```python
from build123d import *

# Parameters (mm, degrees)
ESBO_O1_W                = 120
ESBO_O1_H                = 204
RESSALTO_EXTRUS_O1_DEPTH = 60
ESBO_O2_W                = 114
ESBO_O2_H                = 198
CORTE_EXTRUS_O1_DEPTH    = 57
ESBO_O4_W                = 86
ESBO_O4_H                = 149
CORTE_EXTRUS_O2_DEPTH    = 45
ESBO_O7_W                = 3
ESBO_O7_H                = 204
RESSALTO_EXTRUS_O2_DEPTH = 15
ESBO_O12_W               = 3
ESBO_O12_H               = 204
RESSALTO_EXTRUS_O3_DEPTH = 15
ESBO_O13_W               = 150
ESBO_O13_H               = 3
RESSALTO_EXTRUS_O4_DEPTH = 10
ESBO_O14_W               = 150
ESBO_O14_H               = 3
RESSALTO_EXTRUS_O5_DEPTH = 10
FILETE1_R                = 10
ESBO_O15_W               = 3
ESBO_O15_H               = 5
ESBO_O15_W_2             = 5
ESBO_O15_H_2             = 3
CORTE_EXTRUS_O4_DEPTH    = 5
FILETE2_R                = 10
FILETE3_R                = 10
FILETE4_R                = 10
FILETE5_R                = 2
FILETE6_R                = 2
FILETE8_R                = 2


with BuildPart() as part:
    # Esboço1 → Ressalto-extrusão1 (new body)
    with BuildSketch(Plane.XY):
        with Locations((27.324641181, 48.820153307)):
            Rectangle(ESBO_O1_W, ESBO_O1_H)
    extrude(amount=RESSALTO_EXTRUS_O1_DEPTH)

    # Esboço2 → Corte-extrusão1 (cut)
    with BuildSketch(Plane(origin=(0, 0, 0), x_dir=(-1, 0, 0), z_dir=(0, 0, -1))):
        with Locations((-27.324641181, 48.820153307)):
            Rectangle(ESBO_O2_W, ESBO_O2_H)
    extrude(amount=-CORTE_EXTRUS_O1_DEPTH, mode=Mode.SUBTRACT)

    # Esboço4 → Corte-extrusão2 (cut)
    with BuildSketch(Plane.XY.offset(60)):
        with Locations((27.324641181, 48.820153307)):
            Rectangle(ESBO_O4_W, ESBO_O4_H)
    extrude(amount=-CORTE_EXTRUS_O2_DEPTH, mode=Mode.SUBTRACT)

    # Esboço7 → Ressalto-extrusão2 (add)
    with BuildSketch(Plane(origin=(87.324641181, 0, 0), x_dir=(0, 0, -1), z_dir=(1, 0, 0))):
        with Locations((-58.5, 48.820153307)):
            Rectangle(ESBO_O7_W, ESBO_O7_H)
    extrude(amount=RESSALTO_EXTRUS_O2_DEPTH)

    # Esboço12 → Ressalto-extrusão3 (add)
    with BuildSketch(Plane.ZY.offset(32.675358819)):
        with Locations((58.5, 48.820153307)):
            Rectangle(ESBO_O12_W, ESBO_O12_H)
    extrude(amount=RESSALTO_EXTRUS_O3_DEPTH)

    # Esboço13 → Ressalto-extrusão4 (add)
    with BuildSketch(Plane(origin=(0, 150.820153307, 0), x_dir=(1, 0, 0), z_dir=(0, 1, 0))):
        with Locations((27.324641181, -58.5)):
            Rectangle(ESBO_O13_W, ESBO_O13_H)
    extrude(amount=RESSALTO_EXTRUS_O4_DEPTH)

    # Esboço14 → Ressalto-extrusão5 (add)
    with BuildSketch(Plane.XZ.offset(53.179846693)):
        with Locations((27.324641181, 58.5)):
            Rectangle(ESBO_O14_W, ESBO_O14_H)
    extrude(amount=RESSALTO_EXTRUS_O5_DEPTH)

    # Filete1
    filete1_edges = [part.edges().sort_by_distance(p)[0] for p in [
        (102.324641181, 160.820153307, 58.5),
    ]]
    fillet(filete1_edges, radius=FILETE1_R)

    # Esboço15 → Corte-extrusão4 (cut)
    with BuildSketch(Plane(origin=(0, 0, 0), x_dir=(-1, 0, 0), z_dir=(0, 0, -1))):
        with Locations((31.175358819, 48.820153307)):
            Rectangle(ESBO_O15_W, ESBO_O15_H)
        with Locations((-27.324641181, 149.320153307)):
            Rectangle(ESBO_O15_W_2, ESBO_O15_H_2)
        with Locations((-27.324641181, -51.679846693)):
            Rectangle(ESBO_O15_W_2, ESBO_O15_H_2)
        with Locations((-85.824641181, 48.820153307)):
            Rectangle(ESBO_O15_W, ESBO_O15_H)
    extrude(amount=-CORTE_EXTRUS_O4_DEPTH, mode=Mode.SUBTRACT)

    # Filete2
    filete2_edges = [part.edges().sort_by_distance(p)[0] for p in [
        (-47.675358819, 160.820153307, 58.5),
    ]]
    fillet(filete2_edges, radius=FILETE2_R)

    # Filete3
    filete3_edges = [part.edges().sort_by_distance(p)[0] for p in [
        (102.324641181, -63.179846693, 58.5),
    ]]
    fillet(filete3_edges, radius=FILETE3_R)

    # Filete4
    filete4_edges = [part.edges().sort_by_distance(p)[0] for p in [
        (-47.675358819, -63.179846693, 58.5),
    ]]
    fillet(filete4_edges, radius=FILETE4_R)

    # Filete5
    filete5_edges = [part.edges().sort_by_distance(p)[0] for p in [
        (-32.675358819, -53.179846693, 28.5),
    ]]
    fillet(filete5_edges, radius=FILETE5_R)

    # Filete6
    filete6_edges = [part.edges().sort_by_distance(p)[0] for p in [
        (-32.675358819, 150.820153307, 28.5),
        (87.324641181, 150.820153307, 28.5),
        (87.324641181, -53.179846693, 28.5),
    ]]
    fillet(filete6_edges, radius=FILETE6_R)

    # Filete8
    filete8_edges = [part.edges().sort_by_distance(p)[0] for p in [
        (-15.675358819, 123.320153307, 58.5),
        (70.324641181, 123.320153307, 58.5),
        (70.324641181, -25.679846693, 58.5),
        (-15.675358819, -25.679846693, 58.5),
    ]]
    fillet(filete8_edges, radius=FILETE8_R)


solid = part.part
```
For this review, take the finished solid that the model builds, in its own axes (mm). A direction names the side the tool comes from. Give positions to 0.01 mm unless a question says otherwise; leave off trailing zeros. Write each loop counter-clockwise with the first axis right and the second up, starting at its lowest first coordinate (ties: lowest second). Pieces come first, ordered by that corner, then holes. Notation, with made-up numbers: M 39,29 L 93,29 A26 cw 93,59 Z; hole C 51.25,-26.75 d10. An arc over 180 degrees is marked long. Answer as CSV lines item,"result".
1. Consider section D-D, the plane y = 143.5. Write out the cut boundary in (x, z), then the cut area to 3 significant figures.
Findings:
outline,"M -47.68,57 L -32.68,57 L -32.68,0 L -29.68,0 L -29.68,57 L 84.32,57 L 84.32,0 L 87.32,0 L 87.32,57 L 102.32,57 L 102.32,60 L -47.68,60 Z"
area,"792 mm2"
2. For faces 5 (the flat face through (28, -53.18, 28)), 6 (the flat face through (28, 150.82, 28)), 7 (the flat face through (-32.675, 47, 28)), 8 (the flat face through (87.325, 47, 28)), 9 (the flat face through (-29.675, 47, 28)), list the 3-axis set-ups (+Z, -Z, +X, -X, +Y, -Y) from which the entire face can be reached by the end or side of a thin tool; tool diameter is ignored.
Findings:
face 5,"-Z, +X, -X, -Y"
face 6,"-Z, +X, -X, +Y"
face 7,"-Z, -X, +Y, -Y"
face 8,"-Z, +X, +Y, -Y"
face 9,"-Z"
3. Consider section C-C, the plane y = 63. Write out the cut boundary in (x, z).
Findings:
outline,"M -47.68,57 L -32.68,57 L -32.68,0 L -29.68,0 L -29.68,57 L -15.68,57 L -15.68,60 L -47.68,60 Z; M 70.32,57 L 84.32,57 L 84.32,0 L 87.32,0 L 87.32,57 L 102.32,57 L 102.32,60 L 70.32,60 Z"
4. Wall thickness on line 1 (Y direction, x = 59, z = 39); line 2 (X direction, y = 43.5, z = 35.5); line 3 (Z direction, x = 81, y = 67): over which ranges is each line inside the solid? List them lowest first.
Findings:
line 1,"y = -53.18 to -50.18, 147.82 to 150.82"
line 2,"x = -32.68 to -29.68, 84.32 to 87.32"
line 3,"z = 57 to 60"
5. Draft analysis for pull direction X (two halves, no side actions). For faces 1 (the flat face through (28, 147.82, 28)), 2 (the flat face through (-32, 123, 0)), 3 (the cylindrical face through (99.473, -60.173, 58.521)), 4 (the flat face through (84.325, 47, 28)), state which applies: +X half, -X half, draft (parallel to the pull), parting line (faces both ways), or undercut.
Findings:
face 1,"undercut"
face 2,"draft"
face 3,"+X half"
face 4,"undercut"
6. Consider section B-B, the plane x = 59.5. Write out the cut boundary in (y, z).
Findings:
outline,"M -63.18,57 L -53.18,57 L -53.18,0 L -50.18,0 L -50.18,57 L -25.68,57 L -25.68,60 L -63.18,60 Z; M 123.32,57 L 147.82,57 L 147.82,0 L 150.82,0 L 150.82,57 L 160.82,57 L 160.82,60 L 123.32,60 Z"
7. For pin 1 (2.5 mm diameter, centred on x = 86.5, z = 2, fed in from +Y); pin 2 (10 mm diameter, centred on y = 111.5, z = 50.5, fed in from -X); pin 3 (3.5 mm diameter, centred on x = 85.5, z = 3, fed in from -Y), all flat-tipped, find the tip position at first contact; note any pin that passes through.
Findings:
pin 1,"stops at y = 150.82"
pin 2,"stops at x = -32.68"
pin 3,"stops at y = -53.18"
8. Consider section A-A, the plane z = 32. Write out the cut boundary in (x, y).
Findings:
outline,"M -32.68,-51.18 A2 ccw -30.68,-53.18 L 85.32,-53.18 A2 ccw 87.32,-51.18 L 87.32,148.82 A2 ccw 85.32,150.82 L -30.68,150.82 A2 ccw -32.68,148.82 Z; hole M -29.68,-50.18 L 84.32,-50.18 L 84.32,147.82 L -29.68,147.82 Z"
